from build123d import *

# Parameters (mm, degrees)
SKETCH_4_W      = 52
SKETCH_4_H      = 80
EXTRUDE_3_DEPTH = 3
EXTRUDE_6_DEPTH = 10
EXTRUDE_7_REACH = 51.979
SKETCH_7_W      = 10
SKETCH_7_H      = 1


with BuildPart() as part:
    # 草图4 → 凸台-拉伸3 (new body)
    with BuildSketch(Plane.XY):
        Rectangle(SKETCH_4_W, SKETCH_4_H)
    extrude(amount=-EXTRUDE_3_DEPTH)

    # 草图6 → 凸台-拉伸6 (add)
    with BuildSketch(Plane.XY):
        Polygon((26, 40), (23.978927851, 40), (23.978927851, 39), (25, 39), (25, 38), (26, 38), align=None)
        Polygon((-25, -38), (-26, -38), (-26, -40), (-23.978927851, -40), (-23.978927851, -39), (-25, -39), align=None)
        Polygon((23.978927851, -39), (23.978927851, -40), (26, -40), (26, -38), (25, -38), (25, -39), align=None)
        Polygon((-26, 40), (-26, 38), (-25, 38), (-25, 39), (-23.978927851, 39), (-23.978927851, 40), align=None)
    extrude(amount=EXTRUDE_6_DEPTH)

    # 草图7 → 凸台-拉伸7 (add, up to next)
    with BuildSketch(Plane(origin=(-23.978927851, 0, 0), x_dir=(0, 0, -1), z_dir=(1, 0, 0)), mode=Mode.PRIVATE) as extrude_7_sk1:
        with Locations((-5, -39.5)):
            Rectangle(SKETCH_7_W, SKETCH_7_H)
    extrude_7_tool1 = extrude(extrude_7_sk1.sketch, amount=EXTRUDE_7_REACH, mode=Mode.PRIVATE) - part.part
    add(extrude_7_tool1.solids().sort_by_distance((-23.978928, -39.5, 5))[0])


solid = part.part
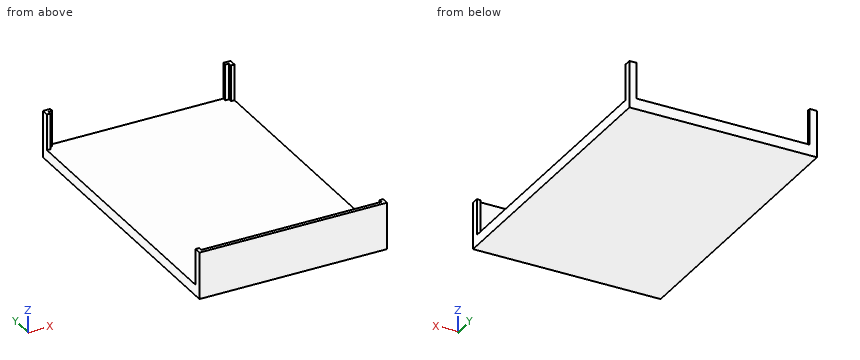
The model under review builds one solid part; all positions refer to its coordinate system, in mm. Round coordinates to 2 decimals unless told otherwise and drop trailing zeros. Write each loop counter-clockwise with the first axis right and the second up, starting at its lowest first coordinate (ties: lowest second). Pieces come first, ordered by that corner, then holes. Notation, with made-up numbers: M -7,-10 L 41,-10 A16 cw 41,-4 Z; hole C 84,88.25 d7. An arc over 180 degrees is marked long. Use a Markdown table: item, result. Add a question column.
Q1. We need section B-B, the plane x = 13.5. State the section outline as (y, z) points, plus the area to 3 significant figures.
Q2. To check wall thickness, follow line 1 (Z direction, x = 11.5, y = -28); line 2 (Y direction, x = -5.5, z = 2.5). State the ranges of each line that lie inside material, in increasing order.
Q3. Insertion check: pin 1 (8 mm diameter, centred on x = -20.5, y = -19.5, fed in from +Z); pin 2 (6 mm diameter, centred on y = -11, z = 4.5, fed in from -X); pin 3 (3 mm diameter, centred on x = -4, z = 5, fed in from +Y). Each pin has a flat end and moves straight along its axis. Give the tip position at first contact, or say it passes through.
Q4. We need section C-C, the plane y = -22. State the section outline as (x, z) points, plus the area to 3 significant figures.
Q5. We need section A-A, the plane z = 4.5. State the section outline as (x, y) points, plus the area to 3 significant figures.
Findings below:
| question | item | result |
|---|---|---|
| 1 | outline | M -40,-3 L 40,-3 L 40,0 L -39,0 L -39,10 L -40,10 Z |
| 1 | area | 250 mm² |
| 2 | line 1 | z = -3 to 0 |
| 2 | line 2 | y = -40 to -39 |
| 3 | pin 1 | stops at z = 0 |
| 3 | pin 2 | passes through |
| 3 | pin 3 | stops at y = -39 |
| 4 | outline | M -26,-3 L 26,-3 L 26,0 L -26,0 Z |
| 4 | area | 156 mm² |
| 5 | outline | M -26,-40 L 26,-40 L 26,-38 L 25,-38 L 25,-39 L -25,-39 L -25,-38 L -26,-38 Z; M -26,38 L -25,38 L -25,39 L -23.98,39 L -23.98,40 L -26,40 Z; M 23.98,39 L 25,39 L 25,38 L 26,38 L 26,40 L 23.98,40 Z |
| 5 | area | 60.0 mm² |
